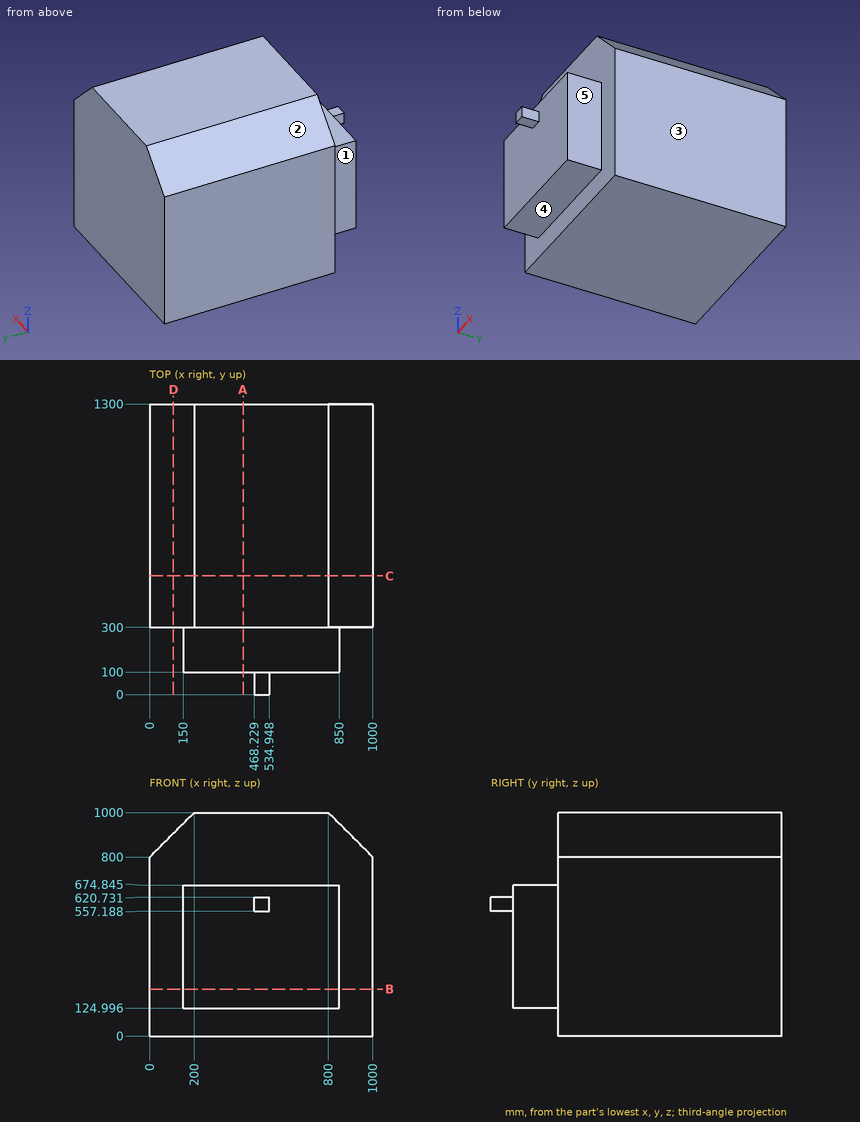
Job drawing, mm, ordinate dimensions from the low corner. One solid piece. A direction names the side the tool comes from. Coordinates: 2 decimals unless noted, no trailing zeros. Loops run counter-clockwise (first coordinate to the right, second up) from the corner with the lowest first, then second, coordinate; pieces in that order, holes last. Notation, with made-up numbers: (-30, 8.5) - (-8, 8.5) arc R9 cw to (-8, 15.5) - close; hole circle Ø4 at (71.25, 89). An arc over 180 degrees is marked (long way). Answer as a JSON object with one key per item and string values. Group by question number.
(1) Probe line 1 along Y through (x, z) = (814, 614); line 2 along Y through (x, z) = (886, 358); line 3 along Z through (x, y) = (548.5, 283) (1 decimal). List the from-to ranges inside material, lowest first.
(2) Flat gauge pins, fed straight in: pin 1 (4 mm diameter, centred on y = 180.5, z = 273.5, fed in from -X); pin 2 (5 mm diameter, centred on x = 341.5, z = 596.5, fed in from -Y); pin 3 (19 mm diameter, centred on y = 33.5, z = 591.5, fed in from -X). Where does each tip first touch, or does it go through?
(3) Tool access for the marked faces 1, 2, 3, 4 and 5: list every direction of +Z, -Z, +X, -X, +Y, -Y with a clear straight run to the whole face (end or side of a thin tool).
(4) Cut at C-C (y = 530.5). Give the cut face in (x, z), then the cut area to 3 significant figures.
(5) Cut at D-D (x = 107). Give the cut face in (y, z).
(6) Cut at A-A (x = 419). Give the cut face in (y, z) (1 decimal).
(7) Cut at B-B (z = 210). Give the cut face in (x, y), then the cut area to 3 significant figures.
Geometry says:
{
 "1": {"line 1": "y = 100 to 1300", "line 2": "y = 300 to 1300", "line 3": "z = 125 to 674.8"},
 "2": {"pin 1": "stops at x = 150", "pin 2": "stops at y = 100", "pin 3": "stops at x = 468.23"},
 "3": {"face 1": "+Z, -Z, -X, -Y", "face 2": "+Z, -X, +Y, -Y", "face 3": "+Z, -Z, +X, +Y, -Y", "face 4": "-Z, +X, -X, -Y", "face 5": "+Z, -Z, +X, -Y"},
 "4": {"outline": "(0, 0) - (1000, 0) - (1000, 800) - (800, 1000) - (200, 1000) - (0, 800) - close", "area": "960,000 mm^2"},
 "5": {"outline": "(300, 0) - (1300, 0) - (1300, 907) - (300, 907) - close"},
 "6": {"outline": "(100, 125) - (300, 125) - (300, 0) - (1300, 0) - (1300, 1000) - (300, 1000) - (300, 674.8) - (100, 674.8) - close"},
 "7": {"outline": "(0, 300) - (150, 300) - (150, 100) - (850, 100) - (850, 300) - (1000, 300) - (1000, 1300) - (0, 1300) - close", "area": "1,140,000 mm^2"}
}
